Geometry check sheet. Reference: the model listing, model coordinates, mm. A direction names the side the tool comes from. Round coordinates to 2 decimals unless told otherwise and drop trailing zeros. Loops run counter-clockwise (first coordinate to the right, second up) from the corner with the lowest first, then second, coordinate; pieces in that order, holes last. Notation, with made-up numbers: (88.5, 55.5) -> (121.5, 55.5) arc R15 ccw to (121.5, 79.5) -> close; hole circle Ø8 at (11, -27.75). An arc over 180 degrees is marked (long way). Use a Markdown table: item, result. Add a question column.
Q1. Gauge pin test, flat ends, axial feed: P1, Ø12, axis at y = -17.5, z = 13, coming from the -X side; P2, Ø5.5, axis at x = -4.5, y = 2, coming from the -Z side; P3, Ø5, axis at x = 18, z = 14, coming from the -Y side; P4, Ø5, axis at x = 22, y = 13, coming from the -Z side. Record the tip position at first contact, or that the pin passes through.
Q2. Sectioned sample at B-B, the plane y = 0. Enter the section's corners in (x, z) (3 decimals).
Q3. Sectioned sample at A-A, the plane z = 13. Enter the section's corners in (x, y), then the cut area to 3 significant figures.
Q4. Release check for a two-part mould opening along X. For faces 1 (the face through (31, 9.76, 13.13)), 2 (the face through (-23, 0, 0)), 3 (the face through (-6, 0, 16)), 4 (the face through (2, -6, 8.5)) record: released by +X, released by -X, zero draft, split by the parting line, or undercut.
Q5. Material ranges on L1, parallel to Y at x = 0, z = 17.25; L2, parallel to Z at x = 16, y = -2.5; L3, parallel to X at y = 10, z = 8.5, recorded low to high.
Q6. Set-up check for faces 5 (the face through (1.172, 8.923, 14.077)), 6 (the face through (0, -6, 26.5)): record each of +Z, -Z, +X, -X, +Y, -Y from which the full face is reachable in a straight line by a thin tool's end or side.
```python
from build123d import *

# Parameters (mm, degrees)
ESBO_O1_R                = 32.5
RESSALTO_EXTRUS_O1_DEPTH = 26.5
ESBO_O2_R                = 22.5
CORTE_EXTRUS_O1_DEPTH    = 23.5
ESBO_O3_R                = 9
RESSALTO_EXTRUS_O2_DEPTH = 15
FILETE1_R                = 4
ESBO_O4_R                = 2.025
CORTE_EXTRUS_O2_DEPTH    = 27.5
FILLET1_R                = 5


with BuildPart() as part:
    # Esboço1 → Ressalto-extrusão1 (new body)
    with BuildSketch(Plane.XY):
        Circle(ESBO_O1_R)
    extrude(amount=RESSALTO_EXTRUS_O1_DEPTH)

    # Esboço2 → Corte-extrusão1 (cut)
    with BuildSketch(Plane(origin=(0, 0, 0), x_dir=(-1, 0, 0), z_dir=(0, 0, -1))):
        Circle(ESBO_O2_R)
    extrude(amount=-CORTE_EXTRUS_O1_DEPTH, mode=Mode.SUBTRACT)

    # Esboço3 → Ressalto-extrusão2 (add)
    with BuildSketch(Plane(origin=(0, 0, 23.5), x_dir=(-1, 0, 0), z_dir=(0, 0, -1))):
        Circle(ESBO_O3_R)
        Polygon((6, -3.464101615), (6, 3.464101615), (0, 6.92820323), (-6, 3.464101615), (-6, -3.464101615), (0, -6.92820323), align=None, mode=Mode.SUBTRACT)
    extrude(amount=RESSALTO_EXTRUS_O2_DEPTH)

    # Filete1
    filete1_edges = [part.edges().sort_by_distance(p)[0] for p in [
        (9, 0, 23.5),
    ]]
    fillet(filete1_edges, radius=FILETE1_R)

    # Esboço4 → Corte-extrusão2 (cut, through all)
    with BuildSketch(Plane.XY.offset(26.5)):
        Circle(ESBO_O4_R)
    extrude(amount=-CORTE_EXTRUS_O2_DEPTH, mode=Mode.SUBTRACT)

    # Fillet1
    fillet1_edges = [part.edges().sort_by_distance(p)[0] for p in [
        (-32.5, 0, 0),
        (-32.5, 0, 26.5),
    ]]
    fillet(fillet1_edges, radius=FILLET1_R)


solid = part.part
```
Values:
| question | item | result |
|---|---|---|
| 1 | P1 | x = -30.4 |
| 1 | P2 | z = 8.5 |
| 1 | P3 | y = -28.57 |
| 1 | P4 | z = 0 |
| 2 | outline | (-32.5, 5) arc R5 ccw to (-27.5, 0) -> (-22.5, 0) -> (-22.5, 23.5) -> (-13, 23.5) arc R4 cw to (-9, 19.5) -> (-9, 8.5) -> (-6, 8.5) -> (-6, 23.5) -> (-2.025, 23.5) -> (-2.025, 26.5) -> (-27.5, 26.5) arc R5 ccw to (-32.5, 21.5) -> close; (2.025, 23.5) -> (6, 23.5) -> (6, 8.5) -> (9, 8.5) -> (9, 19.5) arc R4 cw to (13, 23.5) -> (22.5, 23.5) -> (22.5, 0) -> (27.5, 0) arc R5 ccw to (32.5, 5) -> (32.5, 21.5) arc R5 ccw to (27.5, 26.5) -> (2.025, 26.5) -> close |
| 3 | outline | circle Ø65 at (0, 0); circle Ø18 at (0, 0); hole circle Ø45 at (0, 0); hole (-6, -3.46) -> (0, -6.93) -> (6, -3.46) -> (6, 3.46) -> (0, 6.93) -> (-6, 3.46) -> close |
| 3 | area | 1,860 mm^2 |
| 4 | face 1 | split by the parting line |
| 4 | face 2 | zero draft |
| 4 | face 3 | undercut |
| 4 | face 4 | undercut |
| 5 | L1 | -32.5 to -22.5, -9 to -6.93, 6.93 to 9, 22.5 to 32.5 |
| 5 | L2 | 23.5 to 26.5 |
| 5 | L3 | -30.92 to -20.16, 20.16 to 30.92 |
| 6 | face 5 | -Z |
| 6 | face 6 | +Z, +X, -X, +Y, -Y |
